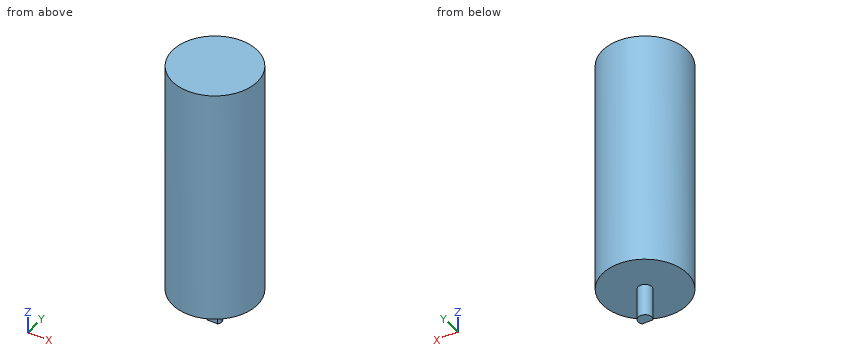
from build123d import *

# Parameters (mm, degrees)
F0_R     = 12.5
F1_DEPTH = 70
F3_DEPTH = 9.5


with BuildPart() as f1:
    # F0 (on Top) → F1 (new body)
    with BuildSketch(Plane.XY):
        Circle(F0_R)
    extrude(amount=F1_DEPTH)

    # F2 (on face) → F3 (join)
    with BuildSketch(Plane(origin=(0, 0, 0), x_dir=(1, 0, 0), z_dir=(0, 0, -1))):
        with BuildLine():
            ThreePointArc((-1.6, 1.2), (-0.632456, -1.897367), (2, 0))
            ThreePointArc((2, 0), (1.897367, 0.632456), (1.6, 1.2))
            Line((1.6, 1.2), (-1.6, 1.2))
        make_face()
    extrude(amount=F3_DEPTH)


solid = f1.part
Read the model definition and answer for the solid it produces. Units are mm, in the model's axes. Give positions to 0.01 mm unless a question says otherwise; leave off trailing zeros. Write each loop counter-clockwise with the first axis right and the second up, starting at its lowest first coordinate (ties: lowest second). Pieces come first, ordered by that corner, then holes. Notation, with made-up numbers: (38.25, 6) - (67.25, 6) arc R20 cw to (67.25, 41) - close; hole circle Ø9 at (74, 28.25). An arc over 180 degrees is marked (long way). Return JSON: item names as keys, results as strings.
Q1. A cutting plane is placed at C-C, the plane y = -2. Determine the outline of the cut face in (x, z), and give its area (3 significant figures).
Reply:
{"outline": "(-12.34, 0) - (12.34, 0) - (12.34, 70) - (-12.34, 70) - close", "area": "1,730 mm²"}
Q2. Given P1, Ø8, axis at y = 6.5, z = 11, coming from the -X side; P2, Ø2, axis at y = 1.5, z = 51, coming from the -X side; P3, Ø1, axis at x = 0, z = -2.5, coming from the -Y side, each flat-ended and moving along its own axis, determine where each tip first touches the part or whether it passes through.
Reply:
{"P1": "x = -12.25", "P2": "x = -12.49", "P3": "y = -1.2"}
Q3. Consider line 1 along Z through (x, y) = (-1, -7); line 2 along X through (y, z) = (2.5, 18.5); line 3 along X through (y, z) = (5, 64). Determine where each line is inside the solid, lowest interval first. Write a range as [from, to].
Reply:
{"line 1": "[0, 70]", "line 2": "[-12.25, 12.25]", "line 3": "[-11.46, 11.46]"}
Q4. A cutting plane is placed at A-A, the plane x = 0. Determine the outline of the cut face in (y, z), and give its area (3 significant figures).
Reply:
{"outline": "(-12.5, 0) - (-1.2, 0) - (-1.2, -9.5) - (2, -9.5) - (2, 0) - (12.5, 0) - (12.5, 70) - (-12.5, 70) - close", "area": "1,780 mm²"}
Q5. A cutting plane is placed at D-D, the plane y = 8.25. Determine the outline of the cut face in (x, z), and give its area (3 significant figures).
Reply:
{"outline": "(-9.39, 0) - (9.39, 0) - (9.39, 70) - (-9.39, 70) - close", "area": "1,310 mm²"}
Q6. A cutting plane is placed at B-B, the plane z = 42.5. Determine the outline of the cut face in (x, y).
Reply:
{"outline": "circle Ø25 at (0, 0)"}
